Part model, mm, in its own coordinate system. Face numbers are marked on the shaded views. A direction names the side the tool comes from. Give positions to 0.01 mm unless a question says otherwise; leave off trailing zeros. Order: outer loops, then holes, each group sorted by start corner. A loop starts at its lowest first (then second) coordinate and runs counter-clockwise, first axis right, second up. Notation, with made-up numbers: (-6.75, 41.5) -> (41.25, 41.5) arc R14 ccw to (41.25, 54.5) -> close; hole circle Ø5 at (71.5, 60.25). An arc over 180 degrees is marked (long way). Write item = value, one per line. Start each with the question number.
Item 1: Band-saw the part on C-C on z = 1.65. Write the cut outline in (x, y) (1 decimal).
Item 2: Band-saw the part on B-B on y = 2.5. Write the cut outline in (x, z), plus the area to 3 significant figures.
Item 3: Drill centre lines: line 1 along Y through (x, z) = (36.83, 2) (3 decimals); line 2 along X through (y, z) = (-0.75, 2.1); line 3 along X through (y, z) = (1, 3.05). Where is each one in solid material? Low to high.
Item 4: Band-saw the part on A-A on x = -36.83. Write the cut outline in (y, z) (3 decimals), plus the area to 3 significant figures.
Item 5: Flat gauge pins, fed straight in: P1, Ø3, axis at x = -27, y = 0.5, coming from the +Z side; P2, Ø1.9, axis at x = 14, y = 1.5, coming from the -Z side; P3, Ø2, axis at x = 36.83, y = 0, coming from the -Z side. Where does each tip first touch, or does it go through?
Item 6: Pull direction X, two halves, no side cores. Call the marked faces 1, 2 and 3: +X half, -X half, draft (parallel to the pull), parting line (faces both ways), or undercut.
Item 7: Band-saw the part on D-D on z = 4.8. Write the cut outline in (x, y) (3 decimals).
Item 8: Tool access for the marked faces 4, 5 and 6: list every direction of +Z, -Z, +X, -X, +Y, -Y with a clear straight run to the whole face (end or side of a thin tool).
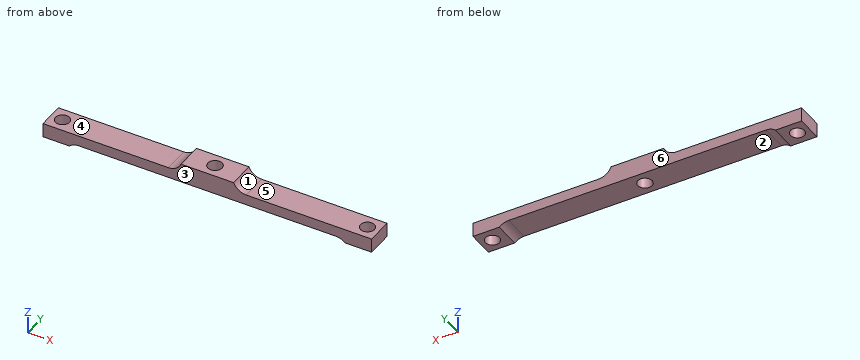
```python
from build123d import *

# Parameters (mm, degrees)
SKETCH1_W             = 79.375
SKETCH1_H             = 6.35
BOSS_EXTRUDE1_DEPTH   = 5.5118
SKETCH10_W            = 66.675
SKETCH10_H            = 6.35
CUT_EXTRUDE2_DEPTH    = 0.89916
SKETCH2_W             = 33.3375
SKETCH2_H             = 6.35
CUT_EXTRUDE1_DEPTH    = 2.07264
M3_CLEARANCE_HOLE1_D  = 3.4
F_8_32_TAPPED_HOLE1_D = 3.4544
FILLET1_R             = 3.302


with BuildPart() as part:
    # Sketch1 → Boss-Extrude1 (new body)
    with BuildSketch(Plane.XY):
        Rectangle(SKETCH1_W, SKETCH1_H)
    extrude(amount=BOSS_EXTRUDE1_DEPTH)

    # Sketch10 → Cut-Extrude2 (cut)
    with BuildSketch(Plane(origin=(0, 0, 0), x_dir=(-1, 0, 0), z_dir=(0, 0, -1))):
        Rectangle(SKETCH10_W, SKETCH10_H)
    extrude(amount=-CUT_EXTRUDE2_DEPTH, mode=Mode.SUBTRACT)

    # Sketch2 → Cut-Extrude1 (cut)
    with BuildSketch(Plane.XY.offset(5.5118)):
        with Locations((23.01875, 0)):
            Rectangle(SKETCH2_W, SKETCH2_H)
    cut_extrude1 = extrude(amount=-CUT_EXTRUDE1_DEPTH, mode=Mode.SUBTRACT)

    # M3 Clearance Hole1 (through all)
    with Locations(Plane.XY.offset(3.43916)):
        with Locations((36.83, 0)):
            m3_clearance_hole1 = Hole(M3_CLEARANCE_HOLE1_D / 2)

    # Mirror2: Cut-Extrude1, M3 Clearance Hole1 across plane
    add(cut_extrude1.mirror(Plane(origin=(0, 0, 0), x_dir=(0, 0, 1), z_dir=(1, 0, 0))), mode=Mode.SUBTRACT)
    add(m3_clearance_hole1.mirror(Plane(origin=(0, 0, 0), x_dir=(0, 0, 1), z_dir=(1, 0, 0))), mode=Mode.SUBTRACT)

    # #8-32 Tapped Hole1 (through all)
    with Locations(Plane.XY.offset(5.5118)):
        with Locations((0, 0)):
            Hole(F_8_32_TAPPED_HOLE1_D / 2)

    # Fillet1
    # the kernel refuses this fillet: 3.302 mm, written as the material it adds along each edge
    with BuildSketch(Plane(origin=(33.3375, 3.175, 0.89916), x_dir=(-1, 0, 0), z_dir=(0, -1, 0))) as fillet1_piece_1:
        with BuildLine():
            CenterArc((2.264854065, 3.302), FILLET1_R, 226.693279333, 43.306720667)
            Line((0, 0.89916), (-0.045297081, 0.8511032))
            ThreePointArc((-0.045297081, 0.8511032), (-0.06604, 0.44958), (-0.06604, 0))
            Line((-0.06604, 0), (0, -0.06604))
            Line((0, -0.06604), (2.264854065, -0.06604))
            Line((2.264854065, -0.06604), (2.264854065, 0))
        make_face()
    extrude(amount=6.35)
    with BuildSketch(Plane(origin=(6.35, 3.175, 3.43916), x_dir=(1, 0, 0), z_dir=(0, -1, 0))) as fillet1_piece_2:
        with BuildLine():
            CenterArc((3.064617103, 3.302), FILLET1_R, 201.858009222, 68.141990778)
            Line((0, 2.07264), (-0.061292342, 2.0480528))
            ThreePointArc((-0.061292342, 2.0480528), (-0.06604, 1.03632), (-0.06604, 0))
            Line((-0.06604, 0), (0, -0.06604))
            Line((0, -0.06604), (3.064617103, -0.06604))
            Line((3.064617103, -0.06604), (3.064617103, 0))
        make_face()
    extrude(amount=6.35)
    with BuildSketch(Plane(origin=(-6.35, 3.175, 3.43916), x_dir=(0, 0, 1), z_dir=(0, -1, 0))) as fillet1_piece_3:
        with BuildLine():
            CenterArc((3.302, 3.064617103), FILLET1_R, 180, 68.141990778)
            Line((0, 3.064617103), (-0.06604, 3.064617103))
            Line((-0.06604, 3.064617103), (-0.06604, 0))
            Line((-0.06604, 0), (0, -0.06604))
            ThreePointArc((0, -0.06604), (1.03632, -0.06604), (2.0480528, -0.061292342))
            Line((2.0480528, -0.061292342), (2.07264, 0))
        make_face()
    extrude(amount=6.35)
    with BuildSketch(Plane(origin=(-33.3375, -3.175, 0.89916), x_dir=(0, 0, -1), z_dir=(0, 1, 0))) as fillet1_piece_4:
        with BuildLine():
            CenterArc((3.302, -2.264854065), FILLET1_R, 136.693279333, 43.306720667)
            Line((0, -2.264854065), (-0.06604, -2.264854065))
            Line((-0.06604, -2.264854065), (-0.06604, 0))
            Line((-0.06604, 0), (0, 0.06604))
            ThreePointArc((0, 0.06604), (0.44958, 0.06604), (0.8511032, 0.045297081))
            Line((0.8511032, 0.045297081), (0.89916, 0))
        make_face()
    extrude(amount=6.35)


solid = part.part
```
Values found:
q1.outline = (-39.7, -3.2) -> (39.7, -3.2) -> (39.7, 3.2) -> (-39.7, 3.2) -> close; hole circle Ø3.4 at (-36.8, 0); hole circle Ø3.5 at (0, 0); hole circle Ø3.4 at (36.8, 0)
q2.outline = (-39.69, 0) -> (-33.34, 0) arc R3.3 cw to (-31.07, 0.9) -> (31.07, 0.9) arc R3.3 cw to (33.34, 0) -> (39.69, 0) -> (39.69, 3.44) -> (9.41, 3.44) arc R3.3 cw to (6.35, 5.51) -> (-6.35, 5.51) arc R3.3 cw to (-9.41, 3.44) -> (-39.69, 3.44) -> close
q2.area = 244 mm^2
q3.line_1 = -3.175 to -1.7, 1.7 to 3.175
q3.line_2 = -39.69 to -38.36, -35.3 to -1.56, 1.56 to 35.3, 38.36 to 39.69
q3.line_3 = -39.69 to -38.2, -35.46 to -1.41, 1.41 to 35.46, 38.2 to 39.69
q4.outline = (-3.175, 0) -> (-1.7, 0) -> (-1.7, 3.439) -> (-3.175, 3.439) -> close; (1.7, 0) -> (3.175, 0) -> (3.175, 3.439) -> (1.7, 3.439) -> close
q4.area = 10.1 mm^2
q5.P1 = 3.44
q5.P2 = 0.9
q5.P3 = through
q6.face_1 = +X half
q6.face_2 = undercut
q6.face_3 = draft
q7.outline = (-6.743, -3.175) -> (6.743, -3.175) -> (6.743, 3.175) -> (-6.743, 3.175) -> close; hole circle Ø3.454 at (0, 0)
q8.face_4 = +Z, -X, +Y, -Y
q8.face_5 = +Z, +X, +Y, -Y
q8.face_6 = +Z, -Z, +X, -X, +Y
